Check sheet for the modelled part. Datum: model origin and axes. Units: mm. Face numbers are marked on the shaded views. Coordinates: 2 decimals unless noted, no trailing zeros. Loops run counter-clockwise (first coordinate to the right, second up) from the corner with the lowest first, then second, coordinate; pieces in that order, holes last. Notation, with made-up numbers: (44.5, 64) - (74.5, 64) arc R12 cw to (74.5, 74) - close; hole circle Ø8 at (18, 43.25). An arc over 180 degrees is marked (long way). Answer as a JSON object with one key per item and string values. Group by question number.
from build123d import *

# Parameters (mm, degrees)
SKETCH1_R           = 26.25
BOSS_EXTRUDE1_DEPTH = 89
CUT_EXTRUDE1_DEPTH  = 8
SKETCH29_W          = 1
SKETCH29_H          = 1.5
CHAMFER1_SIZE       = 2


with BuildPart() as part:
    # Sketch1 → Boss-Extrude1 (new, symmetric)
    with BuildSketch(Plane.XY):
        Circle(SKETCH1_R)
    extrude(amount=BOSS_EXTRUDE1_DEPTH, both=True)

    # Sketch2 → Cut-Extrude1 (cut)
    with BuildSketch(Plane.XY.offset(89)):
        with BuildLine():
            Line((-20.810153772, 16), (20.810153772, 16))
            ThreePointArc((20.810153772, 16), (0, 26.25), (-20.810153772, 16))
        make_face()
        with BuildLine():
            Line((20.810153772, -16), (-20.810153772, -16))
            ThreePointArc((-20.810153772, -16), (0, -26.25), (20.810153772, -16))
        make_face()
    cut_extrude1 = extrude(amount=-CUT_EXTRUDE1_DEPTH, mode=Mode.SUBTRACT)

    # Sketch27 → 1/2-20 Tapped Hole3 (revolve, cut)
    with BuildSketch(Plane(origin=(0, 0, 89), x_dir=(0, -1, 0), z_dir=(1, 0, 0))):
        Polygon((0, 0), (0, 13.45757432), (5.75437, 10), (5.75437, 0), align=None)
    f_1_2_20_tapped_hole3 = revolve(axis=Axis((0, 0, 95.35), (0, 0, -1)), mode=Mode.SUBTRACT)

    # Mirror2: Cut-Extrude1, 1/2-20 Tapped Hole3 across plane
    add(cut_extrude1.mirror(Plane.XY), mode=Mode.SUBTRACT)
    add(f_1_2_20_tapped_hole3.mirror(Plane.XY), mode=Mode.SUBTRACT)

    # Sketch29 → Cut-Revolve1 (revolve, cut)
    with BuildSketch(Plane(origin=(0, 0, 0), x_dir=(1, 0, 0), z_dir=(0, 1, 0)), mode=Mode.PRIVATE) as cut_revolve1_sk:
        with Locations((25.75, 70.25)):
            Rectangle(SKETCH29_W, SKETCH29_H)
    cut_revolve1 = revolve(cut_revolve1_sk.sketch.rotate(Axis((0, 0, 89), (0, 0, -1)), 217.555079253), axis=Axis((0, 0, 89), (0, 0, -1)), mode=Mode.SUBTRACT)

    # Mirror3: Cut-Revolve1 across plane
    add(cut_revolve1.mirror(Plane.XY), mode=Mode.SUBTRACT)

    # Chamfer1
    chamfer1_edges = [part.edges().sort_by_distance(p)[0] for p in [
        (-26.25, 0, -89),
        (24.852857346, -8.449732644, -89),
        (-26.25, 0, 89),
        (24.852857346, 8.449732644, 89),
    ]]
    chamfer(chamfer1_edges, length=CHAMFER1_SIZE)


solid = part.part
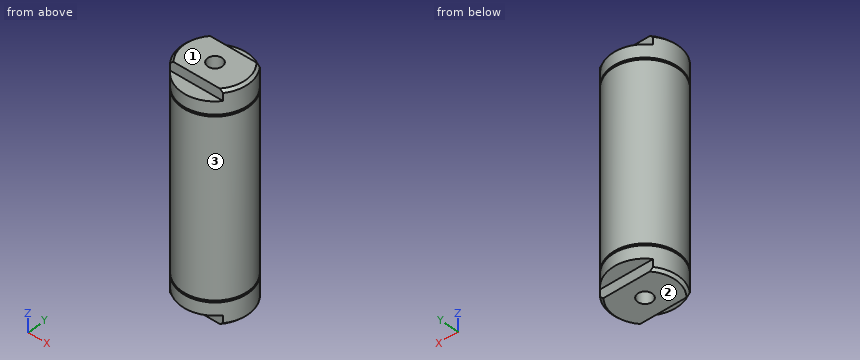
1. Sectioned sample at C-C on z = 24.5. Record the cut outline in (x, y).
2. Gauge pin test, flat ends, axial feed: pin 1 (6.5 mm diameter, centred on x = -6, z = 87, fed in from -Y); pin 2 (1.5 mm diameter, centred on x = -8, z = -8.5, fed in from -Y); pin 3 (3 mm diameter, centred on x = 10, y = 20.5, fed in from -Z). Record the tip position at first contact, or that the pin passes through.
3. Sectioned sample at B-B on x = -13.5. Record the cut outline in (y, z), plus the area to 3 significant figures.
4. Sectioned sample at A-A on y = -18.5. Record the cut outline in (x, z), plus the area to 3 significant figures.
5. Material ranges on line 1 (Z direction, x = 9, y = -24); line 2 (Y direction, x = 0, z = -84.5); line 3 (X direction, y = 0, z = -86.5), recorded low to high.
6. Release check for a two-part mould opening along Z. For the marked faces 1, 2 and 3 record: released by +Z, released by -Z, zero draft, split by the parting line, or undercut.
Answers follow:
{
 "1": {"outline": "circle Ø52.5 at (0, 0)"},
 "2": {"pin 1": "stops at y = -16", "pin 2": "stops at y = -25.23", "pin 3": "stops at z = -81"},
 "3": {"outline": "(-22.51, -81) - (-16, -81) - (-16, -89) - (16, -89) - (16, -81) - (22.51, -81) - (22.51, -71) - (21.34, -71) - (21.34, -69.5) - (22.51, -69.5) - (22.51, 69.5) - (21.34, 69.5) - (21.34, 71) - (22.51, 71) - (22.51, 81) - (16, 81) - (16, 89) - (-16, 89) - (-16, 81) - (-22.51, 81) - (-22.51, 71) - (-21.34, 71) - (-21.34, 69.5) - (-22.51, 69.5) - (-22.51, -69.5) - (-21.34, -69.5) - (-21.34, -71) - (-22.51, -71) - close", "area": "7,800 mm^2"},
 "4": {"outline": "(-18.62, -81) - (18.62, -81) - (18.62, -71) - (17.18, -71) - (17.18, -69.5) - (18.62, -69.5) - (18.62, 69.5) - (17.18, 69.5) - (17.18, 71) - (18.62, 71) - (18.62, 81) - (-18.62, 81) - (-18.62, 71) - (-17.18, 71) - (-17.18, 69.5) - (-18.62, 69.5) - (-18.62, -69.5) - (-17.18, -69.5) - (-17.18, -71) - (-18.62, -71) - close", "area": "6,030 mm^2"},
 "5": {"line 1": "z = -81 to -71, -69.5 to 69.5, 71 to 81", "line 2": "y = -16 to -5.75, 5.75 to 16", "line 3": "x = -26.25 to -5.75, 5.75 to 26.25"},
 "6": {"face 1": "released by +Z", "face 2": "released by -Z", "face 3": "zero draft"}
}
